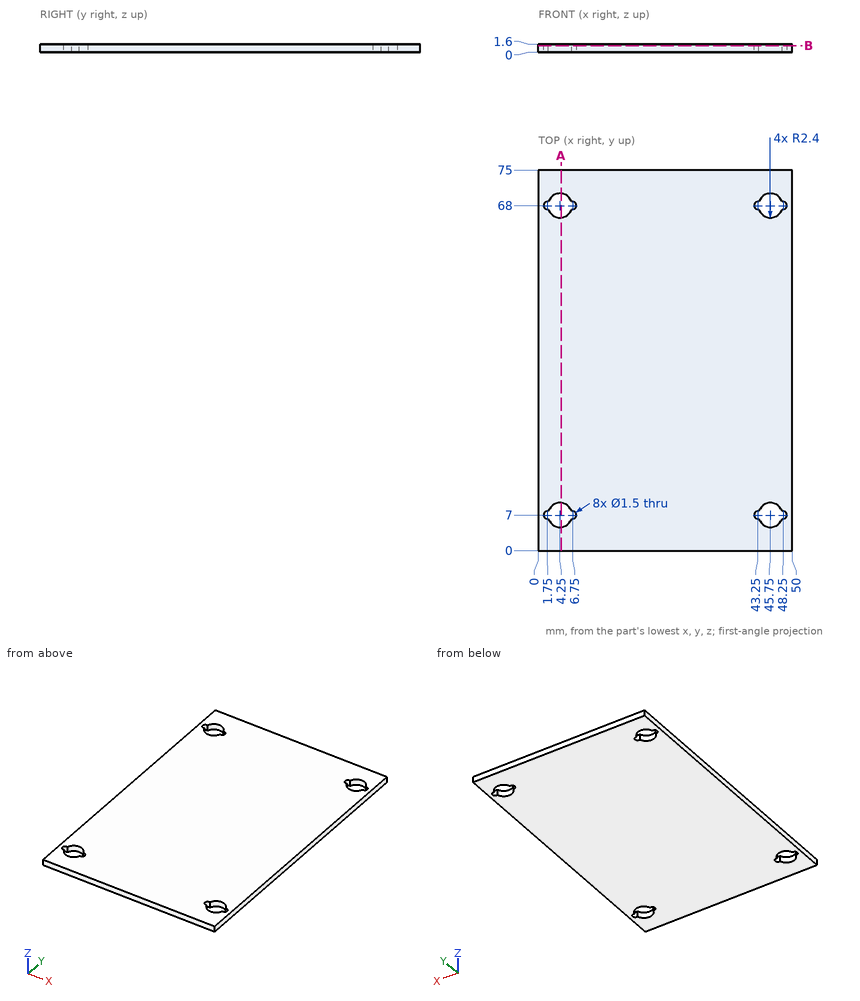
Here's the drawing with two shaded views (mm, measured from the low corner). I have some questions. Coordinates: 2 decimals unless noted, no trailing zeros. Order: outer loops, then holes, each group sorted by start corner. A loop starts at its lowest first (then second) coordinate and runs counter-clockwise, first axis right, second up. Notation, with made-up numbers: (6.5, 24.5) -> (28.5, 24.5) arc R31 ccw to (28.5, 48.5) -> close; hole circle Ø8 at (-22.75, -33). An arc over 180 degrees is marked (long way). One line per question, with ' | ' between items.
Q1. Imagine slicing it at A-A on x = 4.5. Please give me the cut outline in (y, z), and give its area (3 significant figures).
Return value:
outline: (0, 0) -> (4.61, 0) -> (4.61, 1.6) -> (0, 1.6) -> close; (9.39, 0) -> (65.61, 0) -> (65.61, 1.6) -> (9.39, 1.6) -> close; (70.39, 0) -> (75, 0) -> (75, 1.6) -> (70.39, 1.6) -> close | area: 105 mm²
Q2. I'm going to push flat-ended pins straight in: P1, Ø1.2, axis at x = 43.25, y = 68, coming from the -Z side; P2, Ø10, axis at x = 14.5, y = 30, coming from the -Z side. Where does each tip first touch, or does it pass through?
Return value:
P1: through | P2: z = 0
Q3. If I drill on L1, parallel to Y at x = 48.25, z = 0.8; L2, parallel to Y at x = 4, z = 0.8; L3, parallel to X at y = 5.5, z = 0.4, over which ranges is the centre line in solid material (lowest first)?
Return value:
L1: 0 to 6.25, 7.75 to 67.25, 68.75 to 75 | L2: 0 to 4.61, 9.39 to 65.61, 70.39 to 75 | L3: 0 to 2.38, 6.12 to 43.88, 47.62 to 50
Q4. Imagine slicing it at B-B on z = 1.3. Please give me the cut outline in (x, y).
Return value:
outline: (0, 0) -> (50, 0) -> (50, 75) -> (0, 75) -> close; hole (1.96, 6.28) arc R2.4 ccw to (6.54, 6.28) arc R0.75 ccw (long way) to (6.54, 7.72) arc R2.4 ccw to (1.96, 7.72) arc R0.75 ccw (long way) to start; hole (1.96, 67.28) arc R2.4 ccw to (6.54, 67.28) arc R0.75 ccw (long way) to (6.54, 68.72) arc R2.4 ccw to (1.96, 68.72) arc R0.75 ccw (long way) to start; hole (43.46, 6.28) arc R2.4 ccw to (48.04, 6.28) arc R0.75 ccw (long way) to (48.04, 7.72) arc R2.4 ccw to (43.46, 7.72) arc R0.75 ccw (long way) to start; hole (43.46, 67.28) arc R2.4 ccw to (48.04, 67.28) arc R0.75 ccw (long way) to (48.04, 68.72) arc R2.4 ccw to (43.46, 68.72) arc R0.75 ccw (long way) to start
